Answer from the drawing. Dimensions are ordinates in mm from the lowest x, y and z of the part. A direction names the side the tool comes from. Give positions to 0.01 mm unless a question says otherwise; leave off trailing zeros. Loops run counter-clockwise (first coordinate to the right, second up) from the corner with the lowest first, then second, coordinate; pieces in that order, holes last. Notation, with made-up numbers: (-11.5, 11.5) - (4.5, 11.5) arc R16 cw to (4.5, 27.5) - close; hole circle Ø8 at (-13.75, 17). An arc over 180 degrees is marked (long way). One line per item, written item: value.
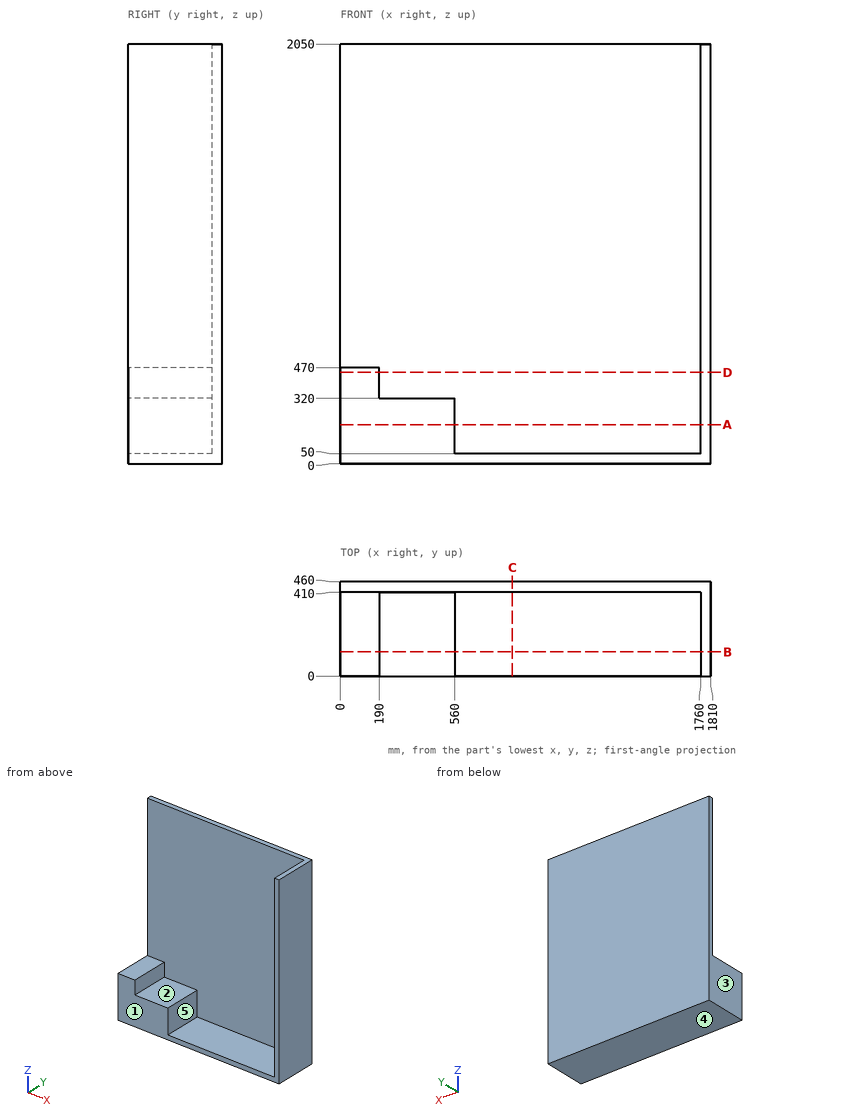
1. The mould has two halves that part along X. Classify the marked faces 3, 4 and 5: released by +X, released by -X, zero draft, split by the parting line, or undercut.
Output:
face 3: released by -X
face 4: zero draft
face 5: undercut
2. Section D-D (z = 447) is taken. Write down the section's boundary in (x, y).
Output:
outline: (0, 0) - (190, 0) - (190, 410) - (1760, 410) - (1760, 0) - (1810, 0) - (1810, 460) - (0, 460) - close
3. Section A-A (z = 191.5) is taken. Write down the section's boundary in (x, y), and give its area (3 significant figures).
Output:
outline: (0, 0) - (560, 0) - (560, 410) - (1760, 410) - (1760, 0) - (1810, 0) - (1810, 460) - (0, 460) - close
area: 341,000 mm²
4. Section B-B (y = 118) is taken. Write down the section's boundary in (x, z).
Output:
outline: (0, 0) - (1810, 0) - (1810, 2050) - (1760, 2050) - (1760, 50) - (560, 50) - (560, 320) - (190, 320) - (190, 470) - (0, 470) - close
5. Flat-ended cylindrical pins translate along their axes: pin 1 Ø6 at (y, z) = (299.5, 1689.5) entering from -X; pin 2 Ø8 at (x, y) = (1189, 234) entering from -Z. Find the tip coordinate at first contact, or state that the pin passes through.
Output:
pin 1: stops at x = 1760
pin 2: stops at z = 0
6. Section C-C (x = 840) is taken. Write down the section's boundary in (y, z).
Output:
outline: (0, 0) - (460, 0) - (460, 2050) - (410, 2050) - (410, 50) - (0, 50) - close
7. For the marked faces 1 and 2, determine the directions among +Z, -Z, +X, -X, +Y, -Y from which every point of the face is accessible in a straight line to the end or side of a thin tool.
Output:
face 1: +Z, -Z, +X, -X, -Y
face 2: +Z, -Y
8. Find the intervals of material crossed by line 1 along X through (y, z) = (92, 92.5); line 2 along X through (y, z) = (384, 1028); line 3 along Z through (x, y) = (587, 239.5), in increasing order.
Output:
line 1: x = 0 to 560, 1760 to 1810
line 2: x = 1760 to 1810
line 3: z = 0 to 50
